from build123d import *

# Parameters (mm, degrees)
BOSS_EXTRUDE1_DEPTH = 20
CUT_EXTRUDE1_DEPTH  = 10
CUT_EXTRUDE2_DEPTH  = 10


with BuildPart() as part:
    # Sketch1 → Boss-Extrude1 (new body)
    with BuildSketch(Plane.XY):
        Polygon((0, 0), (15, 0), (15, 25), (-5, 25), (-5, 15), (-15, 15), align=None)
    extrude(amount=BOSS_EXTRUDE1_DEPTH)

    # Sketch2 → Cut-Extrude1 (cut)
    with BuildSketch(Plane.XY.offset(20)):
        Polygon((5, 25), (5, 0), (0, 0), (-15, 15), (-5, 15), (-5, 25), align=None)
    extrude(amount=-CUT_EXTRUDE1_DEPTH, mode=Mode.SUBTRACT)

    # Sketch3 → Cut-Extrude2 (cut)
    with BuildSketch(Plane.ZY.offset(-5)):
        Polygon((10, 25), (20, 25), (20, 15), align=None)
    extrude(amount=-CUT_EXTRUDE2_DEPTH, mode=Mode.SUBTRACT)


solid = part.part
The model under review builds one solid part; all positions refer to its coordinate system, in mm. A direction names the side the tool comes from. Round coordinates to 2 decimals unless told otherwise and drop trailing zeros. Order: outer loops, then holes, each group sorted by start corner. A loop starts at its lowest first (then second) coordinate and runs counter-clockwise, first axis right, second up. Notation, with made-up numbers: (-28.75, 66) -> (27.25, 66) arc R21 cw to (27.25, 101) -> close; hole circle Ø5 at (-40, 8). An arc over 180 degrees is marked (long way). Use CSV: the item, a comma, the result in double quotes. Start each with the question number.
(1) Consider section C-C on z = 5.25. Write out the cut boundary in (x, y).
(2) Consider section D-D on z = 13. Write out the cut boundary in (x, y).
(3) Consider section B-B on x = 11.5. Write out the cut boundary in (y, z), and give its area (3 significant figures).
(4) Tool access review of faces 1 (the face through (-10, 15, 5)), 2 (the face through (15, 12, 10)), 3 (the face through (5, 10, 15)): name each direction out of +Z, -Z, +X, -X, +Y, -Y from which nothing blocks a thin tool from reaching the whole face with its end or side.
(5) Wall thickness on probe 1 along X at (y, z) = (23.25, 5.5); probe 2 along Z at (x, y) = (-1, 21.5); probe 3 along X at (y, z) = (22.25, 11): over which ranges is each line inside the solid? List them lowest first. Write a range as from..to.
(6) Insertion check: pin 1 (12 mm diameter, centred on y = 22, z = 4.5, fed in from -X); pin 2 (8 mm diameter, centred on y = 15.5, z = 15.5, fed in from -X); pin 3 (5 mm diameter, centred on x = -8.5, z = 10, fed in from +Y); pin 4 (4 mm diameter, centred on x = -8, z = 13, fed in from +Y). Each pin has a flat end and moves straight along its axis. Give the tip position at first contact, or say it passes through.
(7) Consider section A-A on y = 7. Write out the cut boundary in (x, z), and give its area (3 significant figures).
Responses:
1,outline,"(-15, 15) -> (0, 0) -> (15, 0) -> (15, 25) -> (-5, 25) -> (-5, 15) -> close"
2,outline,"(5, 0) -> (15, 0) -> (15, 22) -> (5, 22) -> close"
3,outline,"(0, 0) -> (25, 0) -> (25, 10) -> (15, 20) -> (0, 20) -> close"
3,area,"450 mm²"
4,face 1,"+Z, -Z, -X, +Y"
4,face 2,"+Z, -Z, +X, +Y, -Y"
4,face 3,"+Z, -X, +Y, -Y"
5,probe 1,"-5..15"
5,probe 2,"0..10"
5,probe 3,"5..15"
6,pin 1,"x = -5"
6,pin 2,"x = 5"
6,pin 3,"y = 15"
6,pin 4,"through"
7,outline,"(-7, 0) -> (15, 0) -> (15, 20) -> (5, 20) -> (5, 10) -> (-7, 10) -> close"
7,area,"320 mm²"
